Read the model definition and answer for the solid it produces. Units are mm, in the model's axes. Face numbers are marked on the shaded views. A direction names the side the tool comes from. Coordinates: 2 decimals unless noted, no trailing zeros. Order: outer loops, then holes, each group sorted by start corner. A loop starts at its lowest first (then second) coordinate and runs counter-clockwise, first axis right, second up. Notation, with made-up numbers: (-30, 25) - (-15, 25) arc R15 cw to (-15, 47) - close; hole circle Ø2 at (-39.75, -18). An arc over 180 degrees is marked (long way). Answer as a JSON object with one key per item and string values. Group by question number.
from build123d import *

# Parameters (mm, degrees)
F0_W     = 1200
F0_H     = 250
F1_DEPTH = 15
F2_W     = 1200
F2_H     = 25
F3_DEPTH = 25
F4_W     = 1000
F4_H     = 15
F5_DEPTH = 150


with BuildPart() as f1:
    # F0 (on Front) → F1 (new body)
    with BuildSketch(Plane.XZ):
        Rectangle(F0_W, F0_H)
    extrude(amount=-F1_DEPTH)

    # F2 (on face) → F3 (join)
    with BuildSketch(Plane(origin=(0, 15, 0), x_dir=(-1, 0, 0), z_dir=(0, 1, 0))):
        with Locations((0, 112.5)):
            Rectangle(F2_W, F2_H)
    extrude(amount=F3_DEPTH)

    # F4 (on face) → F5 (join)
    with BuildSketch(Plane(origin=(0, 15, 0), x_dir=(-1, 0, 0), z_dir=(0, 1, 0))):
        with Locations((0, -7.5)):
            Rectangle(F4_W, F4_H)
    extrude(amount=F5_DEPTH)

    # F6: F1 across face


with BuildPart() as f1_1:
    add(f1.part)
    add(f1.part.mirror(Plane(origin=(0, 165, -7.5), x_dir=(-1, 0, 0), z_dir=(0, 1, 0))))


solid = f1_1.part
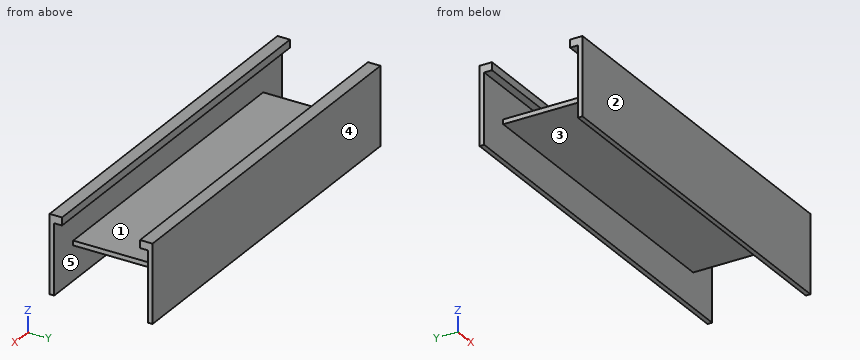
1. Straight lines are drawn through the part: L1, parallel to Z at x = -153, y = 311.5; L2, parallel to Y at x = 267, z = 33.5; L3, parallel to Z at x = -70.5, y = 44. For each, find the intervals that lie inside material, in ascending order.
2. For the marked faces 1 and 2, determine the directions among +Z, -Z, +X, -X, +Y, -Y from which every point of the face is accessible in a straight line to the end or side of a thin tool.
3. A cutting plane is placed at D-D on x = -153. Write down the section's boundary in (y, z), and give its area (4 significant figures).
4. A cutting plane is placed at C-C on y = 145.5. Write down the section's boundary in (x, z), and give its area (3 significant figures).
5. For a pull along Z with two mould halves and no side action, classify the marked faces 3, 4 and 5 as pulls with the +Z half, pulls with the -Z half, needs draft (parallel to the pull), parting line crosses it, or undercut.
6. A cutting plane is placed at B-B on z = 83. Write down the section's boundary in (x, y).
7. A cutting plane is placed at A-A on x = 521.5. Write down the section's boundary in (y, z), and give its area (3 significant figures).
8. Given pin 1 (16.5 mm diameter, centred on y = 193, z = -5, fed in from +X); pin 2 (16.5 mm diameter, centred on y = 151, z = -10.5, fed in from -X); pin 3 (20 mm diameter, centred on x = -288.5, y = 301, fed in from -Z); pin 4 (12.5 mm diameter, centred on x = -124, z = 106.5, fed in from -Y), each flat-ended and moving along its own axis, determine where each tip first touches the part or whether it passes through.
Derived:
{
 "1": {"L1": "z = -15 to 0, 100 to 125", "L2": "y = 0 to 15, 315 to 330", "L3": "z = -15 to 0"},
 "2": {"face 1": "+X, -X", "face 2": "+Z, -Z, +X, -X, -Y"},
 "3": {"outline": "(0, -125) - (15, -125) - (15, -15) - (315, -15) - (315, -125) - (330, -125) - (330, 125) - (290, 125) - (290, 100) - (315, 100) - (315, 0) - (15, 0) - (15, 100) - (40, 100) - (40, 125) - (0, 125) - close", "area": "13,250 mm2"},
 "4": {"outline": "(-500, -15) - (500, -15) - (500, 0) - (-500, 0) - close", "area": "15,000 mm2"},
 "5": {"face 3": "pulls with the -Z half", "face 4": "needs draft", "face 5": "undercut"},
 "6": {"outline": "(-600, 0) - (600, 0) - (600, 15) - (-600, 15) - close; (-600, 315) - (600, 315) - (600, 330) - (-600, 330) - close"},
 "7": {"outline": "(0, -125) - (15, -125) - (15, 100) - (40, 100) - (40, 125) - (0, 125) - close; (290, 100) - (315, 100) - (315, -125) - (330, -125) - (330, 125) - (290, 125) - close", "area": "8,750 mm2"},
 "8": {"pin 1": "stops at x = 500", "pin 2": "stops at x = -500", "pin 3": "stops at z = -15", "pin 4": "stops at y = 0"}
}
